Can you work these out from the drawing? Everything is in mm from the part's minimum corner. Give positions to 0.01 mm unless a question says otherwise; leave off trailing zeros. Loops run counter-clockwise (first coordinate to the right, second up) from the corner with the lowest first, then second, coordinate; pieces in that order, holes last.
Q1. If we section it at C-C (x = 81): Please give me the cut outline in (y, z), plus the area to 4 significant figures.
Q2. Will these pins go through, and if not, where does the flat tip stop? P1, Ø2.5, axis at y = 3, z = 1.5, coming from the +X side; P2, Ø1, axis at x = 113, z = 2, coming from the +Y side; P3, Ø1.5, axis at x = 148.5, z = 2.5, coming from the -Y side.
Q3. If we section it at B-B (z = 2.75): Please give me the cut outline in (x, y).
Q4. I need wall thicknesses on line 1 (X direction, y = 38.5, z = 1.1); line 2 (X direction, y = 70.5, z = 4.3); line 3 (X direction, y = 10, z = 1.8). Which ranges of each line are inside material? Lowest first, please.
Q5. If we section it at D-D (y = 15): Please give me the cut outline in (x, z).
Q6. If we section it at A-A (y = 81): Please give me the cut outline in (x, z).
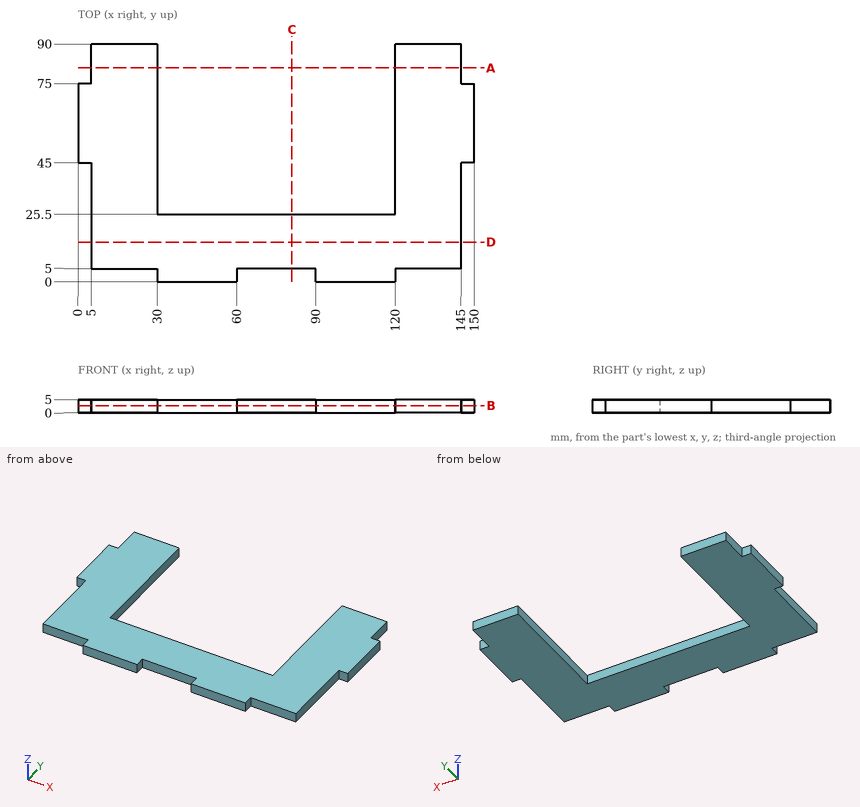
Check sheet entries:
1. outline: (5, 0) - (25.5, 0) - (25.5, 5) - (5, 5) - close
1. area: 102.5 mm2
2. P1: stops at x = 120
2. P2: stops at y = 25.5
2. P3: stops at y = 45
3. outline: (0, 45) - (5, 45) - (5, 5) - (30, 5) - (30, 0) - (60, 0) - (60, 5) - (90, 5) - (90, 0) - (120, 0) - (120, 5) - (145, 5) - (145, 45) - (150, 45) - (150, 75) - (145, 75) - (145, 90) - (120, 90) - (120, 25.5) - (30, 25.5) - (30, 90) - (5, 90) - (5, 75) - (0, 75) - close
4. line 1: x = 5 to 30, 120 to 145
4. line 2: x = 0 to 30, 120 to 150
4. line 3: x = 5 to 145
5. outline: (5, 0) - (145, 0) - (145, 5) - (5, 5) - close
6. outline: (5, 0) - (30, 0) - (30, 5) - (5, 5) - close; (120, 0) - (145, 0) - (145, 5) - (120, 5) - close
